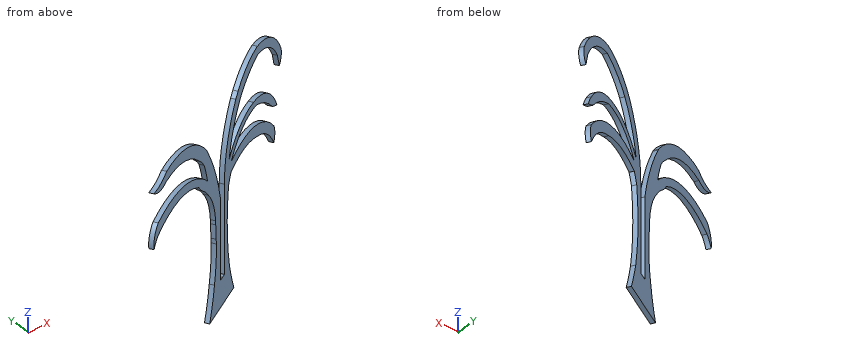
from build123d import *

# Parameters (mm, degrees)
F1_DEPTH = 25.4
F2_ANGLE = 240
F3_ANGLE = 30


# Not quite as in the source:
# - a feature names something its author has since deleted; it is built from what else it names


with BuildPart() as f1:
    # F0 (on Front) → F1 (new body)
    with BuildSketch(Plane.XZ):
        with BuildLine():
            ThreePointArc((250.1826790571, 167.252155113), (278.1130880831, 191.8897284489), (301.4146556953, 220.9440691755))
            ThreePointArc((301.4146556953, 220.9440691755), (548.9344062192, 315.2980350064), (813.1931424143, 296.9672381879))
            ThreePointArc((813.1931424143, 296.9672381879), (843.2368199295, 278.4857074323), (866.6267395021, 252.0830333234))
            ThreePointArc((866.6267395021, 252.0830333234), (859.2886133314, 317.8635284318), (813.1931424141, 365.3622567654))
            ThreePointArc((813.1931424141, 365.3622567654), (528.658381188, 363.1008503302), (268.4933890423, 247.8649133709))
            ThreePointArc((268.4933890423, 247.8649133709), (255.8828799715, 238.6195077853), (243.4818595648, 229.0949523449))
            ThreePointArc((243.4818595648, 229.0949523449), (216.8466348082, 206.3937348312), (191.0419305212, 182.7527172748))
            ThreePointArc((191.0419305212, 182.7527172748), (209.2426753746, 242.3856524278), (234.085008502, 299.5714247227))
            ThreePointArc((234.085008502, 299.5714247227), (262.5639500876, 333.6377098113), (295.1646447182, 363.7832999229))
            ThreePointArc((295.1646447182, 363.7832999229), (301.1050415282, 369.5098935095), (307.1268496022, 375.1508168282))
            ThreePointArc((307.1268496022, 375.1508168282), (495.0303186662, 491.0726231916), (712.7380371094, 527.8003811836))
            ThreePointArc((712.7380371094, 527.8003811836), (794.9345928524, 528.0032351591), (868.764102459, 564.1351938248))
            ThreePointArc((868.764102459, 564.1351938248), (786.3289991041, 561.1323579191), (706.3259482384, 581.2339782715))
            ThreePointArc((706.3259482384, 581.2339782715), (428.7633374116, 531.0006025963), (202.7621120214, 362.2171878815))
            ThreePointArc((202.7621120214, 362.2171878815), (199.8950650536, 358.0887688295), (197.0456982791, 353.9481274337))
            ThreePointArc((197.0456982791, 353.9481274337), (95.8778868485, 174.2465451031), (27.6736820157, -20.3704408073))
            Line((27.6736820157, -20.3704408073), (27.6736820157, -477.5704408073))
            Line((27.6736820157, -477.5704408073), (2.2736820157, -477.5704408073))
            Line((2.2736820157, -477.5704408073), (-23.1156889348, -478.3051807189))
            Line((-23.1156889348, -478.3051807189), (-23.1156889348, -20.3704408073))
            Line((-23.1156889348, -20.3704408073), (-23.1156889348, 23.7159409966))
            ThreePointArc((-23.1156889348, 23.7159409966), (-60.1684665025, 225.1338478784), (-166.475340724, 400.1793563366))
            ThreePointArc((-166.475340724, 400.1793563366), (-181.4907758471, 412.3365760313), (-195.1139737362, 426.0358373953))
            ThreePointArc((-195.1139737362, 426.0358373953), (-309.3402704075, 490.6134334), (-438.5659396648, 513.3870840073))
            ThreePointArc((-438.5659396648, 513.3870840073), (-612.4676441027, 448.3168030455), (-735.3243231773, 309.0969026089))
            ThreePointArc((-735.3243231773, 309.0969026089), (-741.1111301221, 261.6187426822), (-715.9704566002, 220.9295630455))
            ThreePointArc((-715.9704566002, 220.9295630455), (-704.4880158315, 257.5983242076), (-692.3158168793, 294.0439283848))
            ThreePointArc((-692.3158168793, 294.0439283848), (-588.6352200974, 408.0539998704), (-445.0172185898, 463.9273583889))
            ThreePointArc((-445.0172185898, 463.9273583889), (-328.3620257934, 431.1988717022), (-224.5548516512, 368.7196075916))
            ThreePointArc((-224.5548516512, 368.7196075916), (-135.4578046593, 255.1906523593), (-82.276083529, 121.0310012102))
            ThreePointArc((-82.276083529, 121.0310012102), (-222.8986090653, 214.7399937609), (-390.8064365387, 233.7933778763))
            ThreePointArc((-390.8064365387, 233.7933778763), (-534.8506307826, 188.5252288055), (-647.1569538116, 87.6033529639))
            ThreePointArc((-647.1569538116, 87.6033529639), (-668.750342933, 56.6907627964), (-685.8645677567, 23.0906736106))
            ThreePointArc((-685.8645677567, 23.0906736106), (-654.782784529, 37.0530177531), (-625.6527304649, 54.7296761702))
            ThreePointArc((-625.6527304649, 54.7296761702), (-535.9364621749, 135.4019490396), (-429.9600422382, 193.0736303329))
            ThreePointArc((-429.9600422382, 193.0736303329), (-255.1353162114, 185.0540353391), (-107.6677426965, 90.8133143325))
            ThreePointArc((-107.6677426965, 90.8133143325), (-400.8973120765, 91.9617638291), (-647.1569538116, -67.2270804644))
            ThreePointArc((-647.1569538116, -67.2270804644), (-660.0470579155, -114.5363822579), (-647.1569538116, -161.8456840515))
            ThreePointArc((-647.1569538116, -161.8456840515), (-555.302299834, -51.3433620353), (-428.5768360003, 16.3965630051))
            ThreePointArc((-428.5768360003, 16.3965630051), (-268.955549485, 54.7296761702), (-106.0306501957, 34.633411211))
            ThreePointArc((-106.0306501957, 34.633411211), (-89.072951708, 7.7811719553), (-74.492260997, -20.4324727833))
            ThreePointArc((-74.492260997, -20.4324727833), (-58.44709094, -248.3192131796), (-87.0539037033, -474.9719523956))
            ThreePointArc((-87.0539037033, -474.9719523956), (-111.9092602944, -553.3883298655), (-141.9875799101, -629.9534113053))
            Line((-141.9875799101, -629.9534113053), (162.8124200899, -629.9534113053))
            ThreePointArc((162.8124200899, -629.9534113053), (127.6888612329, -543.8827728043), (102.7497877256, -454.3290916329))
            ThreePointArc((102.7497877256, -454.3290916329), (82.6750571268, -348.4939128162), (79.3961640974, -240.8215916548))
            ThreePointArc((79.3961640974, -240.8215916548), (80.2077016296, -226.8972481017), (81.3018441543, -212.9922565991))
            Line((81.3018441543, -212.9922565991), (87.0378738701, -129.2269402374))
            ThreePointArc((87.0378738701, -129.2269402374), (87.6414479673, -117.6100786674), (88.6270669795, -106.0193785337))
            ThreePointArc((88.6270669795, -106.0193785337), (118.4644160965, 4.4171939804), (182.0192138426, 99.534446014))
            ThreePointArc((182.0192138426, 99.534446014), (213.7444570986, 135.7653016553), (250.1826790571, 167.252155113))
        make_face()
        with BuildLine():
            ThreePointArc((290.310142009, 214.3317525479), (290.308974312, 214.3316774306), (290.3078066153, 214.3316023092))
            Line((290.3078066153, 214.3316023092), (290.7207294437, 214.3993956711))
            ThreePointArc((290.7207294437, 214.3993956711), (290.5154263752, 214.3656308704), (290.310142009, 214.3317525479))
        make_face(mode=Mode.SUBTRACT)
    extrude(amount=F1_DEPTH)


with BuildPart() as f1_1:
    # F2: moved
    add(f1.part.rotate(Axis((27.6736820157, -25.4, -248.9704408073), (0, 0, 1)), F2_ANGLE))


with BuildPart() as f1_2:
    # F3: moved
    add(f1_1.part.rotate(Axis((75.0654127471, 5.8848854854, -227.2946198611), (0, 0, -1)), F3_ANGLE))


solid = f1_2.part
The listing builds one solid part. Answer for the finished solid, in the listing's coordinates (mm). Give positions to 0.01 mm unless a question says otherwise; leave off trailing zeros. Use a Markdown table: item, result.
1. Section A-A on x = 318.5 is taken. Count the separate pieces of the cut face and the enclosed holes in it, plus the area to 3 significant figures.
Values follow:
| item | result |
|---|---|
| separate pieces | 3 |
| enclosed holes | 0 |
| area | 4,820 mm² |
2. Find the intervals of material crossed by probe 1 along Z at (x, y) = (-198.5, -141.5); probe 2 along Y at (x, z) = (559, 128); probe 3 along Y at (x, z) = (373.5, 67), in increasing order. Write a range as from..to.
Values follow:
| item | result |
|---|---|
| probe 1 | z = 202.38..261, 357.36..445.38 |
| probe 2 | y = 285.28..314.61 |
| probe 3 | y = 178.19..207.52 |
3. Each of these flat-tipped pins is pushed along its axis until it touches: P1, Ø5, axis at x = 180, z = 96, coming from the +Y side; P2, Ø5, axis at y = 287, z = 94.5, coming from the -X side. Where does it stop, or does it pass through?
Values follow:
| item | result |
|---|---|
| P1 | stops at y = 97.24 |
| P2 | stops at x = 560.02 |
